Autodesk Inventor part; units mm, degrees
ref_plane "YZ Plane" through (0, 0, 0) normal (1, 0, 0) x (0, 1, 0)
ref_plane "XZ Plane" through (0, 0, 0) normal (0, 1, 0) x (-1, 0, 0)
ref_plane "XY Plane" through (0, 0, 0) normal (0, 0, 1) x (1, 0, 0)
sketch "Sketch2" plane through (0, 0, 0) normal (0, 0, 1) x (1, 0, 0)
  line L0 (0, 0) -> (-9.9, 0)
  line L1 (-4.95, 0) -> (-4.95, 2.5)
  line L2 (-4.95, 0) -> (-2.45, 0) construction
  circle A0 centre (-4.95, 5) radius 2.5
  line L3 (-4.95, 7.5) -> (32.05, 7.5) construction
  line L4 (0, 44.5) -> (0, 0)
  line L5 (0, 0) -> (-9.9, 0)
  line L6 (-9.9, 0) -> (-9.9, 44.5)
  line L7 (0, 45.5) -> (0, 0)
  line L8 (0, 0) -> (-9.9, 0)
  line L9 (-9.9, 0) -> (-9.9, 45.5)
  line L10 (-4.95, 7.5) -> (66.05, 7.5) construction
  line L11 (0, 0) -> (-9.9, 0)
  line L12 (-9.9, 0) -> (-9.9, 90)
  line L13 (-9.9, 90) -> (0, 90)
  line L14 (0, 90) -> (0, 0)
  dimension "d35" = 5
  dimension "d33" = 2.5
  dimension "d34" = 90
  dimension "d46" = 9.9
  dimension "d47" = 90
extrude "Extrusion6" add sketch "Sketch2" along normal blind 5
properties part number "Elbow_Cube_Holder_TestFit_V2"
Can you work these out from the model? Positions are in its coordinate system, mm. Coordinates: 2 decimals unless noted, no trailing zeros. Order: outer loops, then holes, each group sorted by start corner. A loop starts at its lowest first (then second) coordinate and runs counter-clockwise, first axis right, second up.
1. If we section it at C-C (z = 3.1): Please give me the cut outline in (x, y), then the cut area to 3 significant figures.
2. I'm going to push a flat-ended pin straight in: pin 1 (3 mm diameter, centred on y = 15, z = 4, fed in from +X). Where does the tip first touch, or does it pass through?
3. Thinking about a two-plate mould opening in Y: for faces 1 (the face through (-5, 90, 2)), 2 (the face through (-5, 46, 5)), 3 (the face through (-5, 0, 2)), 4 (the face through (-2.565, 4.249, 2.465)), which applies, +Y half, -Y half, draft (parallel to the pull), parting line (faces both ways), or undercut?
4. If we section it at A-A (y = 5): Please give me the cut outline in (x, z), then the cut area to 3 significant figures.
5. If we section it at B-B (x = -4.95): Please give me the cut outline in (y, z).
6. I need wall thicknesses on line 1 (X direction, y = 5, z = 3.1); line 2 (Y direction, x = -4.95, z = 2.2); line 3 (Y direction, x = -6, z = 1.5). Which ranges of each line are inside material? Lowest first, please.
Entries:
1. outline: (-9.9, 0) - (0, 0) - (0, 90) - (-9.9, 90) - close; hole circle Ø5 at (-4.95, 5)
1. area: 871 mm2
2. pin 1: stops at x = 0
3. face 1: +Y half
3. face 2: draft
3. face 3: -Y half
3. face 4: undercut
4. outline: (-9.9, 0) - (-7.45, 0) - (-7.45, 5) - (-9.9, 5) - close; (-2.45, 0) - (0, 0) - (0, 5) - (-2.45, 5) - close
4. area: 24.5 mm2
5. outline: (0, 0) - (2.5, 0) - (2.5, 5) - (0, 5) - close; (7.5, 0) - (90, 0) - (90, 5) - (7.5, 5) - close
6. line 1: x = -9.9 to -7.45, -2.45 to 0
6. line 2: y = 0 to 2.5, 7.5 to 90
6. line 3: y = 0 to 2.73, 7.27 to 90
